Check sheet for the modelled part. Datum: model origin and axes. Units: mm. Coordinates: 2 decimals unless noted, no trailing zeros. Loops run counter-clockwise (first coordinate to the right, second up) from the corner with the lowest first, then second, coordinate; pieces in that order, holes last. Notation, with made-up numbers: (-35, 31.25) -> (6, 31.25) arc R10 ccw to (6, 44.25) -> close; hole circle Ø8 at (82, 27). An arc over 180 degrees is marked (long way). Use CSV: the item, a comma, the result in double quotes. Start each with the question number.
1. Sectioned sample at D-D, the plane x = 16. Record the cut outline in (y, z).
2. Release check for a two-part mould opening along Y. For faces 1 (the face through (-0.867, 11.905, -0.14)), 2 (the face through (-15, 12, 0)), 3 (the face through (0, 15, -10)) record: pulls with the +Y half, pulls with the -Y half, needs draft (parallel to the pull), parting line crosses it, or undercut.
3. Thickness scan on L1, parallel to Y at x = 0, z = 1; L2, parallel to Y at x = 1, z = 8.5; L3, parallel to X at y = 8, z = -2.75. Record the ranges inside material, lowest first.
4. Gauge pin test, flat end, axial feed: pin 1 (5 mm diameter, centred on x = 0, y = 8, fed in from +Z) (3 decimals). Record the tip position at first contact, or that the pin passes through.
5. Sectioned sample at A-A, the plane x = 0. Record the cut outline in (y, z).
6. Sectioned sample at C-C, the plane y = 9. Record the cut outline in (x, z).
7. Sectioned sample at B-B, the plane z = 0. Record the cut outline in (x, y).
Autodesk Inventor part; units mm, degrees
ref_plane "YZ Plane" through (0, 0, 0) normal (1, 0, 0) x (0, 1, 0)
ref_plane "XZ Plane" through (0, 0, 0) normal (0, 1, 0) x (-1, 0, 0)
ref_plane "XY Plane" through (0, 0, 0) normal (0, 0, 1) x (1, 0, 0)
sketch "Эскиз1" plane through (0, 0, 0) normal (0, 0, 1) x (1, 0, 0)
  line L0 (-10, 0) -> (10, 0)
  line L1 (-20, 24) -> (20, 24)
  line L2 (20, 24) -> (10, 0)
  line L3 (-10, 0) -> (-20, 24)
  circle A0 centre (0, 8) radius 4
  line L4 (-20, 24) -> (-20, 30)
  line L5 (-20, 30) -> (20, 30)
  line L6 (20, 30) -> (20, 24)
  line L7 (-5.2413, 8) -> (5.4825, 8)
  point P0 (0, 0)
  dimension "d0" = 20
  dimension "d1" = 40
  dimension "d3" = 8
  dimension "d5" = 24
  dimension "d6" = 6
  dimension "d7" = 16
extrude "Выдавливание1" add sketch "Эскиз1" along normal mid plane 20 contours L3 L1 L2 L0
properties part number "2"
Completed:
1,outline,"(14.4, -10) -> (24, -10) -> (24, 10) -> (14.4, 10) -> close"
2,face 1,"undercut"
2,face 2,"pulls with the -Y half"
2,face 3,"needs draft"
3,L1,"0 to 4, 12 to 24"
3,L2,"0 to 4.13, 11.87 to 24"
3,L3,"-13.33 to -4, 4 to 13.33"
4,pin 1,"through"
5,outline,"(0, -10) -> (4, -10) -> (4, 10) -> (0, 10) -> close; (12, -10) -> (24, -10) -> (24, 10) -> (12, 10) -> close"
6,outline,"(-13.75, -10) -> (-3.87, -10) -> (-3.87, 10) -> (-13.75, 10) -> close; (3.87, -10) -> (13.75, -10) -> (13.75, 10) -> (3.87, 10) -> close"
7,outline,"(-20, 24) -> (-10, 0) -> (10, 0) -> (20, 24) -> close; hole circle Ø8 at (0, 8)"
